Part model, mm, in its own coordinate system. Face numbers are marked on the shaded views. A direction names the side the tool comes from. Coordinates: 2 decimals unless noted, no trailing zeros. Write each loop counter-clockwise with the first axis right and the second up, starting at its lowest first coordinate (ties: lowest second). Pieces come first, ordered by that corner, then holes. Notation, with made-up numbers: (75, 10.25) -> (117, 10.25) arc R23 cw to (117, 44.25) -> close; hole circle Ø7 at (37.25, -13). An arc over 180 degrees is marked (long way). Write item = value, one per line. Start each with the question number.
Q1. Pin check, flat tips, straight feed: P1, Ø4, axis at x = 18.5, y = -67.5, coming from the +Z side; P2, Ø8, axis at x = -41.5, y = -25, coming from the +Z side; P3, Ø8, axis at y = -71.5, z = -30, coming from the -X side. Stop position of each tip, or through.
Q2. Band-saw the part on A-A, the plane x = -22.5. List the corners of the cut face in (y, z).
Q3. Probe line 1 (Y direction, x = -45, z = -8); line 2 (Y direction, x = -6.5, z = -27); line 3 (X direction, y = -84, z = -8). List the from-to ranges inside material, lowest first.
Q4. Band-saw the part on C-C, the plane y = -97. List the corners of the cut face in (x, z), plus the area to 3 significant figures.
Q5. Band-saw the part on D-D, the plane x = 21. List the corners of the cut face in (y, z), plus the area to 3 significant figures.
Q6. Tool access for the marked faces 4, 5, 6 and 7: list every direction of +Z, -Z, +X, -X, +Y, -Y with a clear straight run to the whole face (end or side of a thin tool).
Q7. Band-saw the part on B-B, the plane z = -2.5. List the corners of the cut face in (x, y), plus the area to 3 significant figures.
Q8. Pull direction Y, two halves, no side cores. Call the marked faces 1, 2 and 3: released by +Y, released by -Y, zero draft, split by the parting line, or undercut.
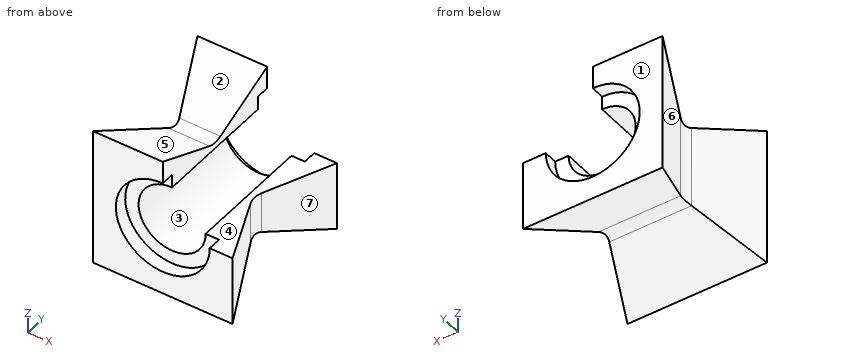
from build123d import *

# Parameters (mm, degrees)
ESQUISSE1_W                  = 104
ESQUISSE1_H                  = 104
BOSS_EXTRU_2_DEPTH           = 56
BOSS_EXTRU_2_DRAFT           = -23
SYM_TRIE1_COPY_1_SKETCH_W    = 104
SYM_TRIE1_COPY_1_SKETCH_H    = 104
SYM_TRIE1_COPY_1_DEPTH       = 56
SYM_TRIE1_COPY_1_DRAFT       = -23
ENL_V_MAT_EXTRU_1_DEPTH      = 134.985073796
ENL_V_MAT_EXTRU_1_DEPTH_BACK = 134.985073796
ESQUISSE2_R                  = 25
CONG_1_R                     = 15
ESQUISSE3_W                  = 52
ESQUISSE3_H                  = 52
ENL_V_MAT_EXTRU_2_DEPTH      = 134.985073796
ESQUISSE4_R                  = 35
ENL_V_MAT_EXTRU_3_DEPTH      = 10


with BuildPart() as part:
    # Esquisse1 → Boss.-Extru.2 (with draft: the straight prism first)
    with BuildSketch(Plane(origin=(0, 0, 0), x_dir=(1, 0, 0), z_dir=(0, 1, 0))):
        Rectangle(ESQUISSE1_W, ESQUISSE1_H)
    extrude(amount=-BOSS_EXTRU_2_DEPTH)
    # Boss.-Extru.2: the draft: its side faces are tilted about the plane it starts from
    boss_extru_2_sides = [part.faces().sort_by_distance(p)[0] for p in [
        (-52, -28, 0),
        (0, -28, 52),
        (52, -28, 0),
        (0, -28, -52),
    ]]
    draft(boss_extru_2_sides, Plane(origin=(0, 0, 0), x_dir=(1, 0, 0), z_dir=(0, 1, 0)), BOSS_EXTRU_2_DRAFT)


with BuildPart() as sym_trie1_copy_1_tool:
    # Symétrie1 copy 1 sketch → Symétrie1 copy 1 (with draft: the straight prism first)
    with BuildSketch(Plane.XZ.offset(112)):
        Rectangle(SYM_TRIE1_COPY_1_SKETCH_W, SYM_TRIE1_COPY_1_SKETCH_H)
    extrude(amount=-SYM_TRIE1_COPY_1_DEPTH)
    # Symétrie1 copy 1: the draft: its side faces are tilted about the plane it starts from
    sym_trie1_copy_1_sides = [sym_trie1_copy_1_tool.faces().sort_by_distance(p)[0] for p in [
        (-52, -84, 0),
        (0, -84, 52),
        (52, -84, 0),
        (0, -84, -52),
    ]]
    draft(sym_trie1_copy_1_sides, Plane.XZ.offset(112), SYM_TRIE1_COPY_1_DRAFT)


with BuildPart() as part_1:
    add(part.part)

    # Symétrie1 copy 1: add sym_trie1_copy_1_tool
    add(sym_trie1_copy_1_tool.part)

    # Esquisse2 → Enlèv. mat.-Extru.1 (cut, two sides: drawn at the far end of the back side and taken through both)
    with BuildSketch(Plane(origin=(0, 0, 0), x_dir=(1, 0, 0), z_dir=(0, 1, 0)).offset(-ENL_V_MAT_EXTRU_1_DEPTH_BACK)):
        with Locations(Location((0, 0, 0), (0, 0, 270))):
            Circle(ESQUISSE2_R)
    extrude(amount=ENL_V_MAT_EXTRU_1_DEPTH + ENL_V_MAT_EXTRU_1_DEPTH_BACK, mode=Mode.SUBTRACT)

    # Congé1
    cong_1_edges = [part_1.edges().sort_by_distance(p)[0] for p in [
        (-28.229410292, -56, 0),
        (0, -56, 28.229410292),
        (28.229410292, -56, 0),
        (0, -56, -28.229410292),
    ]]
    fillet(cong_1_edges, radius=CONG_1_R)

    # Esquisse3 → Enlèv. mat.-Extru.2 (cut, through all)
    with BuildSketch(Plane(origin=(0, 0, 0), x_dir=(1, 0, 0), z_dir=(0, 1, 0))):
        with Locations((26, -26)):
            Rectangle(ESQUISSE3_W, ESQUISSE3_H)
    extrude(amount=-ENL_V_MAT_EXTRU_2_DEPTH, mode=Mode.SUBTRACT)

    # Esquisse4 → Enlèv. mat.-Extru.3 (cut)
    with BuildSketch(Plane(origin=(0, 0, 0), x_dir=(1, 0, 0), z_dir=(0, 1, 0))):
        Circle(ESQUISSE4_R)
    enl_v_mat_extru_3 = extrude(amount=-ENL_V_MAT_EXTRU_3_DEPTH, mode=Mode.SUBTRACT)

    # Symétrie2: Enlèv. mat.-Extru.3 across plane
    add(enl_v_mat_extru_3.mirror(Plane.ZX.offset(-56)), mode=Mode.SUBTRACT)


solid = part_1.part
Ans:
q1.P1 = -14.31
q1.P2 = 43.09
q1.P3 = -36.51
q2.outline = (-112, -52) -> (-61.86, -30.72) arc R15 cw to (-50.14, -30.72) -> (0, -52) -> (0, -26.81) -> (-10, -26.81) -> (-10, -10.9) -> (-102, -10.9) -> (-102, -26.81) -> (-112, -26.81) -> close; (-112, 26.81) -> (-102, 26.81) -> (-102, 10.9) -> (-10, 10.9) -> (-10, 26.81) -> (0, 26.81) -> (0, 52) -> (-50.14, 30.72) arc R15 cw to (-61.86, 30.72) -> (-112, 52) -> close
q3.line_1 = -112 to -95.51, -16.49 to 0
q3.line_2 = -102 to -10
q3.line_3 = -40.11 to -23.69, 23.69 to 40.11
q4.outline = (-45.63, -45.63) -> (45.63, -45.63) -> (45.63, 0) -> (25, 0) arc R25 cw (long way) to (0, 25) -> (0, 45.63) -> (-45.63, 45.63) -> close
q4.area = 4,770 mm2
q5.outline = (-112, -52) -> (-61.86, -30.72) arc R15 cw to (-50.14, -30.72) -> (0, -52) -> (0, -28) -> (-10, -28) -> (-10, -13.56) -> (-102, -13.56) -> (-102, -28) -> (-112, -28) -> close
q5.area = 2,690 mm2
q6.face_4 = +Z, +X, +Y, -Y
q6.face_5 = +Z, +X, -X
q6.face_6 = +Z, -Z, -X
q6.face_7 = +Z, -Z, +X
q7.outline = (-52, -112) -> (-34.91, -112) -> (-34.91, -102) -> (-24.87, -102) -> (-24.87, -10) -> (-34.91, -10) -> (-34.91, 0) -> (-52, 0) -> (-30.72, -50.14) arc R15 cw to (-30.72, -61.86) -> close; (24.87, -102) -> (34.91, -102) -> (34.91, -112) -> (52, -112) -> (30.72, -61.86) arc R15 cw to (30.72, -50.14) -> (52, 0) -> (34.91, 0) -> (34.91, -10) -> (24.87, -10) -> close
q7.area = 3,020 mm2
q8.face_1 = released by +Y
q8.face_2 = undercut
q8.face_3 = zero draft
